Build history of the part. All positions in model axes, mm. Round coordinates to 2 decimals unless told otherwise and drop trailing zeros. Loops run counter-clockwise (first coordinate to the right, second up) from the corner with the lowest first, then second, coordinate; pieces in that order, holes last. Notation, with made-up numbers: (4, 58.25) - (18, 58.25) arc R27 cw to (18, 92.25) - close; hole circle Ø4 at (-12, 30). An arc over 180 degrees is marked (long way). Use one line per item in the form item = value. Start each with the question number.
Q1. Saw through at D-D (z = 3.05). Count the separate pieces of the cut face and the enclosed holes in it, then the cut area to 3 significant figures.
Q2. Saw through at A-A (y = 19.05). Give the cut face in (x, z).
Q3. Drill centre lines: line 1 (Y direction, x = 6.35, z = 3.4); line 2 (Y direction, x = -19.05, z = 1.65); line 3 (X direction, y = 35, z = 3.2). Where is each one in solid material? Low to high.
Q4. Saw through at B-B (x = -19.05). Give the cut face in (y, z).
Q5. Saw through at C-C (y = 31). Give the cut face in (x, z).
Q6. Mould opens along X. For faces 1 (the face through (10.79, 1.81, 2.86)), 2 (the face through (-48.99, 1.91, 2.86)), 3 (the face through (-34.5, 19.72, 2.94)) say: released by +X, released by -X, zero draft, split by the parting line, or undercut.
Q7. Pin check, flat tip, straight feed: pin 1 (5 mm diameter, centred on x = -41, y = 5, fed in from -Z). Stop position of the tip, or through.
```python
from build123d import *

# Parameters (mm, degrees)
SKETCH1_W                = 38.1
SKETCH1_H                = 38.1
BOSS_EXTRUDE1_DEPTH      = 5.8
SKETCH2_R                = 8
CUT_EXTRUDE1_DEPTH       = 12.7
SKETCH3_R                = 1.13
CUT_EXTRUDE2_DEPTH       = 55.19280395
SKETCH4_R                = 0.79375
CUT_EXTRUDE3_DEPTH       = 55.19280395
SKETCH5_W                = 12.7
SKETCH5_H                = 38.1
BOSS_EXTRUDE2_DEPTH      = 5.8
M3_CLEARANCE_HOLE1_D     = 3.4
M3_CLEARANCE_HOLE1_DEPTH = 10
M3_CLEARANCE_HOLE1_TIP   = 1.021463052
SKETCH9_R                = 0.79375
CUT_EXTRUDE4_DEPTH       = 64.764331722
FILLET1_R                = 6.35


with BuildPart() as part:
    # Sketch1 → Boss-Extrude1 (new body)
    with BuildSketch(Plane.XY):
        with Locations((-19.05, 19.05)):
            Rectangle(SKETCH1_W, SKETCH1_H)
    extrude(amount=BOSS_EXTRUDE1_DEPTH)

    # Sketch2 → Cut-Extrude1 (cut)
    with BuildSketch(Plane.XY.offset(5.8)):
        with Locations((-19.05, 19.05)):
            Circle(SKETCH2_R)
    extrude(amount=-CUT_EXTRUDE1_DEPTH, mode=Mode.SUBTRACT)

    # Sketch3 → Cut-Extrude2 (cut, through all)
    with BuildSketch(Plane.XY.offset(5.8)):
        with Locations((-34.925, 34.925)):
            Circle(SKETCH3_R)
        with Locations((-3.175, 34.925)):
            Circle(SKETCH3_R)
        with Locations((-3.175, 3.175)):
            Circle(SKETCH3_R)
        with Locations((-34.925, 3.175)):
            Circle(SKETCH3_R)
    extrude(amount=-CUT_EXTRUDE2_DEPTH, mode=Mode.SUBTRACT)

    # Sketch4 → Cut-Extrude3 (cut, through all)
    with BuildSketch(Plane.XY.offset(5.8)):
        with Locations((-34.925, 19.05)):
            Circle(SKETCH4_R)
        with Locations((-19.05, 34.925)):
            Circle(SKETCH4_R)
        with Locations((-3.175, 19.05)):
            Circle(SKETCH4_R)
        with Locations((-19.05, 3.175)):
            Circle(SKETCH4_R)
    extrude(amount=-CUT_EXTRUDE3_DEPTH, mode=Mode.SUBTRACT)

    # Sketch5 → Boss-Extrude2 (add, through all)
    with BuildSketch(Plane.XY.offset(5.8)):
        with Locations((-44.45, 19.05)):
            Rectangle(SKETCH5_W, SKETCH5_H)
        with Locations((6.35, 19.05)):
            Rectangle(SKETCH5_W, SKETCH5_H)
    extrude(amount=-BOSS_EXTRUDE2_DEPTH)

    # M3 Clearance Hole1
    with Locations(Plane(origin=(0, 0, 0), x_dir=(-1, 0, 0), z_dir=(0, 0, -1))):
        with Locations((-6.35, 31.75), (44.45, 31.75), (44.45, 6.35), (-6.35, 6.35)):
            Hole(M3_CLEARANCE_HOLE1_D / 2, depth=M3_CLEARANCE_HOLE1_DEPTH)
            with Locations((0, 0, -(M3_CLEARANCE_HOLE1_DEPTH + M3_CLEARANCE_HOLE1_TIP / 2))):  # 118° drill point
                Cone(0, M3_CLEARANCE_HOLE1_D / 2, M3_CLEARANCE_HOLE1_TIP, mode=Mode.SUBTRACT)

    # Sketch9 → Cut-Extrude4 (cut, through all)
    with BuildSketch(Plane(origin=(0, 0, 0), x_dir=(-1, 0, 0), z_dir=(0, 0, -1))):
        with Locations((-6.35, 19.05)):
            Circle(SKETCH9_R)
        with Locations((44.45, 19.05)):
            Circle(SKETCH9_R)
    extrude(amount=-CUT_EXTRUDE4_DEPTH, mode=Mode.SUBTRACT)

    # Fillet1
    fillet1_edges = [part.edges().sort_by_distance(p)[0] for p in [
        (-50.8, 0, 2.9),
        (-50.8, 38.1, 2.9),
        (12.7, 38.1, 2.9),
        (12.7, 0, 2.9),
    ]]
    fillet(fillet1_edges, radius=FILLET1_R)


solid = part.part
```
Report:
q1.separate_pieces = 1
q1.enclosed_holes = 15
q1.area = 2,120 mm²
q2.outline = (-50.8, 0) - (-45.24, 0) - (-45.24, 5.8) - (-50.8, 5.8) - close; (-43.66, 0) - (-35.72, 0) - (-35.72, 5.8) - (-43.66, 5.8) - close; (-34.13, 0) - (-27.05, 0) - (-27.05, 5.8) - (-34.13, 5.8) - close; (-11.05, 0) - (-3.97, 0) - (-3.97, 5.8) - (-11.05, 5.8) - close; (-2.38, 0) - (5.56, 0) - (5.56, 5.8) - (-2.38, 5.8) - close; (7.14, 0) - (12.7, 0) - (12.7, 5.8) - (7.14, 5.8) - close
q3.line_1 = 0 to 4.65, 8.05 to 18.26, 19.84 to 30.05, 33.45 to 38.1
q3.line_2 = 0 to 2.38, 3.97 to 11.05, 27.05 to 34.13, 35.72 to 38.1
q3.line_3 = -49.91 to -36.05, -33.8 to -19.84, -18.26 to -4.3, -2.05 to 11.81
q4.outline = (0, 0) - (2.38, 0) - (2.38, 5.8) - (0, 5.8) - close; (3.97, 0) - (11.05, 0) - (11.05, 5.8) - (3.97, 5.8) - close; (27.05, 0) - (34.13, 0) - (34.13, 5.8) - (27.05, 5.8) - close; (35.72, 0) - (38.1, 0) - (38.1, 5.8) - (35.72, 5.8) - close
q5.outline = (-50.8, 0) - (-45.98, 0) - (-45.98, 5.8) - (-50.8, 5.8) - close; (-42.92, 0) - (4.82, 0) - (4.82, 5.8) - (-42.92, 5.8) - close; (7.88, 0) - (12.7, 0) - (12.7, 5.8) - (7.88, 5.8) - close
q6.face_1 = released by +X
q6.face_2 = released by -X
q6.face_3 = undercut
q7.pin_1 = 0
